Could you check a few things on this model? Use its own coordinates, in mm. A direction names the side the tool comes from. Round coordinates to 2 decimals unless told otherwise and drop trailing zeros. Loops run counter-clockwise (first coordinate to the right, second up) from the corner with the lowest first, then second, coordinate; pieces in that order, holes last.
from build123d import *

# Parameters (mm, degrees)
SKETCH1_W               = 254
SKETCH1_H               = 31.75
BOSS_EXTRUDE1_DEPTH     = 50.8
CUT_EXTRUDE1_DEPTH      = 261.968776868
CUT_EXTRUDE1_DEPTH_BACK = 261.968776868
CUT_EXTRUDE2_DEPTH      = 261.968776868
CUT_EXTRUDE2_DEPTH_BACK = 101.6
CUT_EXTRUDE3_START      = -31.75
CUT_EXTRUDE3_DEPTH      = 31.75
CUT_EXTRUDE4_DEPTH      = 203.2
LPATTERN1_COUNT         = 2
LPATTERN1_PITCH         = 22.86
LPATTERN1_COL_COUNT     = 2
LPATTERN1_COL_PITCH     = 22.86
BOSS_EXTRUDE2_DEPTH     = 12.7
M5_TAPPED_HOLE1_D       = 4.2
M5_TAPPED_HOLE1_DEPTH   = 13.97
M5_TAPPED_HOLE1_TIP     = 1.2618073
FILLET1_R               = 2.54
FILLET2_R               = 5.08


# Read off the part's stored shape, not the designer's step: Cut-Extrude3
with BuildPart() as part:
    # Sketch1 → Boss-Extrude1 (new, symmetric)
    with BuildSketch(Plane.XY):
        with Locations((127, 15.875)):
            Rectangle(SKETCH1_W, SKETCH1_H)
    extrude(amount=BOSS_EXTRUDE1_DEPTH, both=True)

    # Sketch2 → Cut-Extrude1 (cut, two sides: drawn at the far end of the back side and taken through both)
    with BuildSketch(Plane.XY.offset(-CUT_EXTRUDE1_DEPTH_BACK)):
        Polygon((63.5, 31.75), (254, 0), (254, 31.75), align=None)
    extrude(amount=CUT_EXTRUDE1_DEPTH + CUT_EXTRUDE1_DEPTH_BACK, mode=Mode.SUBTRACT)

    # Sketch3 → Cut-Extrude2 (cut, two sides: drawn at the far end of the back side and taken through both)
    with BuildSketch(Plane(origin=(0, 0, 0), x_dir=(1, 0, 0), z_dir=(0, 1, 0)).offset(-CUT_EXTRUDE2_DEPTH_BACK)):
        with BuildLine():
            Line((17.78, 12.7), (17.78, 72.102848299))
            Line((17.78, 72.102848299), (-32.844059738, 72.102848299))
            Line((-32.844059738, 72.102848299), (-31.340021966, -58.533575325))
            Line((-31.340021966, -58.533575325), (17.78, -58.533575325))
            Line((17.78, -58.533575325), (17.78, -12.7))
            ThreePointArc((17.78, -12.7), (11.200161386, -10.734596536), (5.08, -7.62))
            ThreePointArc((5.08, -7.62), (3.005283766, -5.884716234), (1.27, -3.81))
            ThreePointArc((1.27, -3.81), (0.317306771, -2.010897743), (0, 0))
            ThreePointArc((0, 0), (0.317306771, 2.010897743), (1.27, 3.81))
            ThreePointArc((1.27, 3.81), (3.005283766, 5.884716234), (5.08, 7.62))
            ThreePointArc((5.08, 7.62), (11.200161386, 10.734596536), (17.78, 12.7))
        make_face()
    extrude(amount=CUT_EXTRUDE2_DEPTH + CUT_EXTRUDE2_DEPTH_BACK, mode=Mode.SUBTRACT)

    # Cut-Extrude3 outline → Cut-Extrude3 (cut)
    with BuildSketch(Plane(origin=(0, 31.75, 0), x_dir=(1, 0, 0), z_dir=(0, 1, 0)).offset(CUT_EXTRUDE3_START)):
        with BuildLine():
            Line((17.78, 12.7), (62.23, 25.4))
            ThreePointArc((62.23, 25.4), (90.202906045, 37.788778117), (119.38, 46.99))
            ThreePointArc((119.38, 46.99), (133.798896157, 49.763850575), (148.445575226, 50.8))
            Line((148.445575226, 50.8), (17.78, 50.8))
            Line((17.78, 50.8), (17.78, 12.7))
        make_face()
        with BuildLine():
            Line((255, 50.8), (237.800096312, 50.8))
            ThreePointArc((237.800096312, 50.8), (242.634955157, 48.613990909), (246.531625641, 45.012539127))
            ThreePointArc((246.531625641, 45.012539127), (250.977042308, 34.38284899), (254, 23.264676093))
            Line((254, 23.264676093), (255, 18.335620452))
            Line((255, 18.335620452), (255, 50.8))
        make_face()
    cut_extrude3 = extrude(amount=CUT_EXTRUDE3_DEPTH, mode=Mode.SUBTRACT)

    # Mirror2: Cut-Extrude3 across plane
    add(cut_extrude3.mirror(Plane.XY), mode=Mode.SUBTRACT)

    # Sketch7 → Cut-Extrude4 (cut)
    with BuildSketch(Plane(origin=(292.1, 0, 0), x_dir=(0, 0, -1), z_dir=(1, 0, 0))):
        Polygon((-6.35, 24.967833991), (6.35, 24.967833991), (0, 4.647833991), align=None)
    cut_extrude4 = extrude(amount=-CUT_EXTRUDE4_DEPTH, mode=Mode.SUBTRACT)

    # LPattern1: Cut-Extrude4 ×2
    with Locations(*[(0, 0, i * LPATTERN1_PITCH) for i in range(1, LPATTERN1_COUNT)]):
        add(cut_extrude4, mode=Mode.SUBTRACT)

    # LPattern1 col: Cut-Extrude4 ×2
    with Locations(*[(0, 0, -i * LPATTERN1_COL_PITCH) for i in range(1, LPATTERN1_COL_COUNT)]):
        add(cut_extrude4, mode=Mode.SUBTRACT)

    # Sketch9 → Boss-Extrude2 (add)
    with BuildSketch(Plane(origin=(0, 0, 0), x_dir=(0, 0, -1), z_dir=(1, 0, 0))):
        with BuildLine():
            add(Edge.make_bspline(
                [(-25.4, 15.875), (0, 41.275), (25.4, 15.875)],
                knots=[0, 0, 0, 1, 1, 1], degree=2))
            add(Edge.make_bspline(
                [(25.4, 15.875), (0, -9.525), (-25.4, 15.875)],
                knots=[0, 0, 0, 1, 1, 1], degree=2))
        make_face()
    extrude(amount=BOSS_EXTRUDE2_DEPTH)

    # M5 Tapped Hole1
    with Locations(Plane.ZY):
        with Locations((17.78, 15.875), (-17.78, 15.875)):
            Hole(M5_TAPPED_HOLE1_D / 2, depth=M5_TAPPED_HOLE1_DEPTH)
            with Locations((0, 0, -(M5_TAPPED_HOLE1_DEPTH + M5_TAPPED_HOLE1_TIP / 2))):  # 118° drill point
                Cone(0, M5_TAPPED_HOLE1_D / 2, M5_TAPPED_HOLE1_TIP, mode=Mode.SUBTRACT)

    # Fillet1
    fillet1_edges = [part.edges().sort_by_distance(p)[0] for p in [
        (12.7, 15.875, 11.298246193),
        (12.7, 15.875, -11.298246193),
    ]]
    fillet(fillet1_edges, radius=FILLET1_R)

    # Fillet2
    fillet2_edges = [part.edges().sort_by_distance(p)[0] for p in [
        (6.35, 15.875, -25.4),
        (6.35, 15.875, 25.4),
    ]]
    fillet(fillet2_edges, radius=FILLET2_R)


solid = part.part
Item 1: For faces 1 (the flat face through (88.9, 17, 0)), 2 (the flat face through (38, 31.75, 0)), 3 (the flat face through (39.69, 15.65, 18.96)), 4 (the flat face through (39.69, 15.65, -18.96)), which set-ups out of +Z, -Z, +X, -X, +Y, -Y let a thin tool reach every point of the face, with its end or its side?
Results list:
face 1: +X
face 2: +Z, -Z, +X, -X, +Y
face 3: +Z, +Y, -Y
face 4: -Z, +Y, -Y
Item 2: We'd pull the mould along Z, two halves only. Please class faces 5 (the flat face through (12.7, 18, 19)), 6 (the flat face through (143.221, 12.408, 2.425)), 7 (the flat face through (88.9, 17, 23)), 8 (the flat face through (183, 7, 50.8)): released by +Z, released by -Z, zero draft, split by the parting line, or undercut.
Results list:
face 5: zero draft
face 6: undercut
face 7: undercut
face 8: released by +Z
Item 3: Will these pins go through, and if not, where does the flat tip stop? pin 1 (3 mm diameter, centred on x = 100, y = 5.5, fed in from +Z); pin 2 (4 mm diameter, centred on x = 40.5, y = 4.5, fed in from +Z); pin 3 (1 mm diameter, centred on y = 18, z = 26.5, fed in from -X).
Results list:
pin 1: stops at z = 41.78
pin 2: stops at z = 19.76
pin 3: stops at x = 63.41
Item 4: If we section it at B-B, the plane z = 33: Please give me the cut outline in (x, y), then the cut area to 3 significant figures.
Results list:
outline: (78.37, 0) - (251.44, 0) - (251.44, 0.43) - (78.37, 29.27) - close
area: 2,570 mm2
Item 5: If I drill on line 1 along Z through (x, y) = (152.5, 16.5); line 2 along Z through (x, y) = (140.5, 10); line 3 along Y through (x, z) = (10.25, 17.78) (3 decimals), over which ranges is the centre line in solid material (lowest first)?
Results list:
line 1: z = -50.8 to -26.56, -19.16 to -3.7, 3.7 to 19.16, 26.56 to 50.8
line 2: z = -50.46 to -24.53, -21.19 to -1.67, 1.67 to 21.19, 24.53 to 50.46
line 3: y = 9.398 to 13.775, 17.975 to 22.352
Item 6: If we section it at A-A, the plane x = 166: Please give me the cut outline in (y, z).
Results list:
outline: (0, -50.8) - (14.67, -50.8) - (14.67, -25.99) - (4.65, -22.86) - (14.67, -19.73) - (14.67, -3.13) - (4.65, 0) - (14.67, 3.13) - (14.67, 19.73) - (4.65, 22.86) - (14.67, 25.99) - (14.67, 50.8) - (0, 50.8) - close
Item 7: If we section it at C-C, the plane x = 56.5: Please give me the cut outline in (y, z), then the cut area to 3 significant figures.
Results list:
outline: (0, -23.76) - (31.75, -23.76) - (31.75, 23.76) - (0, 23.76) - close
area: 1,510 mm2
